```python
from build123d import *

# Parameters (mm, degrees)
SKETCH_1_R      = 3.35
SKETCH_1_R_2    = 1.5
EXTRUDE_1_DEPTH = 4
SKETCH_3_R      = 1.5
EXTRUDE_2_DEPTH = 13


with BuildPart() as part:
    # 草图1 → 凸台-拉伸1 (new body)
    with BuildSketch(Plane.XY):
        Circle(SKETCH_1_R)
        Circle(SKETCH_1_R_2, mode=Mode.SUBTRACT)
    extrude(amount=EXTRUDE_1_DEPTH)

    # 草图3 → 凸台-拉伸2 (add)
    with BuildSketch(Plane.XY.offset(4)):
        Polygon((3.551375818, -1.681818945), (3.23218584, 2.234672205), (-0.319189978, 3.916491149), (-3.551375818, 1.681818945), (-3.23218584, -2.234672205), (0.319189978, -3.916491149), align=None)
        Circle(SKETCH_3_R, mode=Mode.SUBTRACT)
    extrude(amount=EXTRUDE_2_DEPTH)


solid = part.part
```
Source: CAD feature listing. Evaluate the final solid. Frame: model axes, mm. Coordinates: 2 decimals unless noted, no trailing zeros. Loops run counter-clockwise (first coordinate to the right, second up) from the corner with the lowest first, then second, coordinate; pieces in that order, holes last. Notation, with made-up numbers: M -10,68 L 28,68 A13 cw 28,81 Z; hole C 5,53 d5. An arc over 180 degrees is marked long. Use CSV: the item, a comma, the result in double quotes.
(1) Cut plane C-C on x = 0.75. Return loops of the section in (y, z).
Answers follow:
outline,"M -3.62,4 L -3.26,4 L -3.26,0 L -1.3,0 L -1.3,17 L -3.62,17 Z; M 1.3,0 L 3.26,0 L 3.26,4 L 3.41,4 L 3.41,17 L 1.3,17 Z"
(2) Cut plane A-A on y = -1.25. Return loops of the section in (x, z).
Answers follow:
outline,"M -3.31,4 L -3.11,4 L -3.11,0 L -0.83,0 L -0.83,17 L -3.31,17 Z; M 0.83,0 L 3.11,0 L 3.11,4 L 3.52,4 L 3.52,17 L 0.83,17 Z"
(3) Cut plane D-D on x = 2.5. Return loops of the section in (y, z).
Answers follow:
outline,"M -2.41,4 L -2.23,4 L -2.23,0 L 2.23,0 L 2.23,4 L 2.58,4 L 2.58,17 L -2.41,17 Z"
(4) Draft query along Y for faces 1 (the face through (3, 2, 4)), 2 (the face through (-3.347, 0.147, 1.972)), 3 (the face through (1.913, -2.815, 10.409)), 4 (the face through (-1.5, 0.07, 8.38)). Return one class per face: pulls with the +Y half, pulls with the -Y half, needs draft (parallel to the pull), parting line crosses it, or undercut.
Answers follow:
face 1,"needs draft"
face 2,"parting line crosses it"
face 3,"pulls with the -Y half"
face 4,"undercut"
(5) Cut plane B-B on z = 14. Return loops of the section in (x, y), and give its area (3 significant figures).
Answers follow:
outline,"M -3.55,1.68 L -3.23,-2.23 L 0.32,-3.92 L 3.55,-1.68 L 3.23,2.23 L -0.32,3.92 Z; hole C 0,0 d3"
area,"33.0 mm²"
(6) Line query: line 1 (Y direction, x = 0, z = 8); line 2 (Y direction, x = -1.25, z = 15.25); line 3 (X direction, y = -0.5, z = 2). Output: solid intervals per line, ascending. Write a range as [from, to].
Answers follow:
line 1,"[-3.77, -1.5], [1.5, 3.77]"
line 2,"[-3.17, -0.83], [0.83, 3.27]"
line 3,"[-3.31, -1.41], [1.41, 3.31]"
(7) Contact query for flat-ended pins moving along their axis: pin 1 (1.5 mm diameter, centred on y = -0.5, z = 9, fed in from +X); pin 2 (1 mm diameter, centred on y = -3, z = 7.5, fed in from +X). Output: stop coordinate, or through.
Answers follow:
pin 1,"x = 3.52"
pin 2,"x = 2.37"
